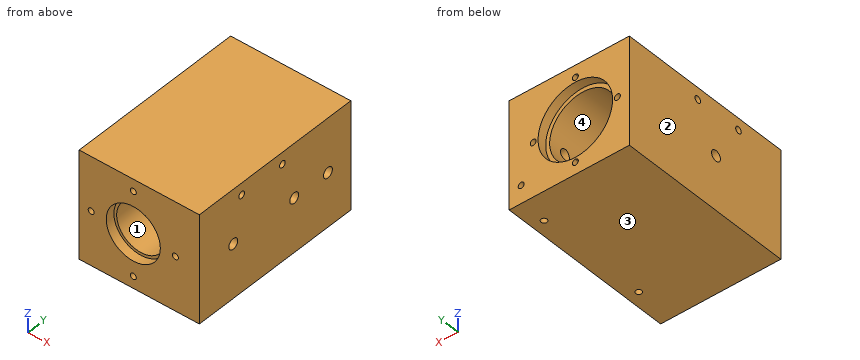
from build123d import *

# Parameters (mm, degrees)
F0_W      = 114.3
F0_H      = 114.3
F1_DEPTH  = 189.13856
F2_R      = 35.179
F3_DEPTH  = 96.52
F4_R      = 39.37
F5_DEPTH  = 9.525
F6_R      = 25.654
F7_DEPTH  = 71.12
F8_R      = 28.575
F9_DEPTH  = 9.525
F10_R     = 7.14375
F11_DEPTH = 118.01956
F12_R     = 5.55625
F13_DEPTH = 32.1059246971
F14_R     = 5.55625
F15_DEPTH = 52.6608720395
F16_DEPTH = 12.7
F18_R     = 3.175
F20_DEPTH = 52.6234315755
F19_R     = 3.175
F21_DEPTH = 146.7612
F24_DEPTH = 9.525
F25_R     = 3.175
F26_DEPTH = 9.525
F27_R     = 3.4925
F28_DEPTH = 127.0010001


with BuildPart() as f1:
    # F0 (on Front) → F1 (new body)
    with BuildSketch(Plane.XZ):
        Rectangle(F0_W, F0_H)
    extrude(amount=F1_DEPTH)

    # F2 (on face) → F3 (cut)
    with BuildSketch(Plane(origin=(0, 0, 0), x_dir=(-1, 0, 0), z_dir=(0, 1, 0))):
        Circle(F2_R)
    extrude(amount=-F3_DEPTH, mode=Mode.SUBTRACT)

    # F4 (on face) → F5 (cut)
    with BuildSketch(Plane(origin=(0, 0, 0), x_dir=(-1, 0, 0), z_dir=(0, 1, 0))):
        Circle(F4_R)
    extrude(amount=-F5_DEPTH, mode=Mode.SUBTRACT)

    # F6 (on face) → F7 (cut)
    with BuildSketch(Plane.XZ.offset(189.13856)):
        Circle(F6_R)
    extrude(amount=-F7_DEPTH, mode=Mode.SUBTRACT)

    # F8 (on face) → F9 (cut)
    with BuildSketch(Plane.XZ.offset(189.13856)):
        Circle(F8_R)
    extrude(amount=-F9_DEPTH, mode=Mode.SUBTRACT)

    # F10 (on face) → F11 (cut, through all)
    with BuildSketch(Plane.XZ.offset(118.01856)):
        Circle(F10_R)
    extrude(amount=-F11_DEPTH, mode=Mode.SUBTRACT)

    # F12 (on face) → F13 (cut, through all)
    with BuildSketch(Plane.YZ.offset(57.15)):
        with Locations((-146.80692, 0)):
            Circle(F12_R)
        with Locations((-70.69328, 0)):
            Circle(F12_R)
        with Locations((-28.575, 0)):
            Circle(F12_R)
    extrude(amount=-F13_DEPTH, mode=Mode.SUBTRACT)

    # F14 (on face) → F15 (cut, through all)
    with BuildSketch(Plane(origin=(-57.15, 0, 0), x_dir=(0, -1, 0), z_dir=(-1, 0, 0))):
        with Locations((108.17606, 0)):
            Circle(F14_R)
    extrude(amount=-F15_DEPTH, mode=Mode.SUBTRACT)

    # F16 (add): a face of the model
    f16_faces = [f1.faces().sort_by_distance(p)[0] for p in [
        (57.15, -94.7404141206, 0),
    ]]
    extrude(f16_faces, amount=F16_DEPTH)

    # F18 (on face) → F20 (cut, through all)
    with BuildSketch(Plane(origin=(0, 0, -57.15), x_dir=(1, 0, 0), z_dir=(0, 0, -1))):
        with Locations((57.15, 146.7612)):
            Circle(F18_R)
        with Locations((57.15, 28.575)):
            Circle(F18_R)
    extrude(amount=-F20_DEPTH, mode=Mode.SUBTRACT)

    # F19 (on face) → F21 (cut)
    with BuildSketch(Plane(origin=(0, 0, 0), x_dir=(-1, 0, 0), z_dir=(0, 1, 0))):
        with Locations((-57.15, -38.1)):
            Circle(F19_R)
    extrude(amount=-F21_DEPTH, mode=Mode.SUBTRACT)

    # F23 (on face) → F24 (cut)
    with BuildSketch(Plane.XZ):
        with BuildLine():
            ThreePointArc((-47.625, 0), (-44.45, -3.175), (-41.275, 0))
            Line((-41.275, 0), (-47.625, 0))
        make_face()
        with BuildLine():
            Line((-47.625, 0), (-41.275, 0))
            ThreePointArc((-41.275, 0), (-44.45, 3.175), (-47.625, 0))
        make_face()
        with BuildLine():
            ThreePointArc((41.275, 0), (44.45, -3.175), (47.625, 0))
            Line((47.625, 0), (41.275, 0))
        make_face()
        with BuildLine():
            Line((41.275, 0), (47.625, 0))
            ThreePointArc((47.625, 0), (44.45, 3.175), (41.275, 0))
        make_face()
        with BuildLine():
            ThreePointArc((0, -41.275), (-3.175, -44.45), (0, -47.625))
            Line((0, -47.625), (0, -41.275))
        make_face()
        with BuildLine():
            Line((0, -41.275), (0, -47.625))
            ThreePointArc((0, -47.625), (2.2450640303, -46.6950640303), (3.175, -44.45))
            ThreePointArc((3.175, -44.45), (2.2450640303, -42.2049359697), (0, -41.275))
        make_face()
        with BuildLine():
            ThreePointArc((0, 47.625), (-3.175, 44.45), (0, 41.275))
            Line((0, 41.275), (0, 47.625))
        make_face()
        with BuildLine():
            Line((0, 47.625), (0, 41.275))
            ThreePointArc((0, 41.275), (2.2450640303, 42.2049359697), (3.175, 44.45))
            ThreePointArc((3.175, 44.45), (2.2450640303, 46.6950640303), (0, 47.625))
        make_face()
    extrude(amount=F24_DEPTH, mode=Mode.SUBTRACT)

    # F25 (on face) → F26 (cut)
    with BuildSketch(Plane.XZ.offset(189.13856)):
        with Locations((-44.45, 0)):
            Circle(F25_R)
        with Locations((0, 44.45)):
            Circle(F25_R)
        with Locations((44.45, 0)):
            Circle(F25_R)
        with Locations((0, -44.45)):
            Circle(F25_R)
    extrude(amount=-F26_DEPTH, mode=Mode.SUBTRACT)

    # F27 (on face) → F28 (cut, through all)
    with BuildSketch(Plane.YZ.offset(69.85)):
        with Locations((-136.2554430962, 44.5877164602)):
            Circle(F27_R)
        with Locations((-85.4554430962, 44.5877164602)):
            Circle(F27_R)
    extrude(amount=-F28_DEPTH, mode=Mode.SUBTRACT)


solid = f1.part
The listing builds one solid part. Answer for the finished solid, in the listing's coordinates (mm). Face numbers are marked on the shaded views. Give positions to 0.01 mm unless a question says otherwise; leave off trailing zeros. Write each loop counter-clockwise with the first axis right and the second up, starting at its lowest first coordinate (ties: lowest second). Pieces come first, ordered by that corner, then holes. Notation, with made-up numbers: (2, -39.75) -> (21, -39.75) arc R5 ccw to (21, -33.75) -> close; hole circle Ø2 at (35, 60.5). An arc over 180 degrees is marked (long way). Use a Markdown table: item, result.
(1) Section B-B, the plane x = -22.5 is taken. Give the number of separate pieces and of enclosed holes in the cut face, then the cut area to 3 significant figures.
Return value:
| item | result |
|---|---|
| separate pieces | 1 |
| enclosed holes | 3 |
| area | 14,300 mm2 |
(2) Determine the mould class of the marked faces 1, 2, 3 and 4 for opening direction X: released by +X, released by -X, zero draft, split by the parting line, or undercut.
Return value:
| item | result |
|---|---|
| face 1 | undercut |
| face 2 | released by -X |
| face 3 | zero draft |
| face 4 | undercut |
(3) Section C-C, the plane z = 32 is taken. Determine the outline of the cut face in (x, y) (3 decimals).
Return value:
| item | result |
|---|---|
| outline | (-57.15, -189.139) -> (69.85, -189.139) -> (69.85, 0) -> (22.935, 0) -> (22.935, -9.525) -> (14.614, -9.525) -> (14.614, -96.52) -> (-14.614, -96.52) -> (-14.614, -9.525) -> (-22.935, -9.525) -> (-22.935, 0) -> (-57.15, 0) -> close |
(4) Section D-D, the plane y = -129.5 is taken. Determine the outline of the cut face in (x, z) (3 decimals), then the cut area to 3 significant figures.
Return value:
| item | result |
|---|---|
| outline | (-57.15, -57.15) -> (69.85, -57.15) -> (69.85, 57.15) -> (-57.15, 57.15) -> close; hole circle Ø51.308 at (0, 0); hole circle Ø6.35 at (57.15, -38.1) |
| area | 12,400 mm2 |
(5) Find the intervals of material crossed by probe 1 along Z at (x, y) = (0, -186) (3 decimals); probe 2 along Y at (x, z) = (57.15, -27.5); probe 3 along Z at (x, y) = (64.5, -147), in increasing order. Write a range as from..to.
Return value:
| item | result |
|---|---|
| probe 1 | -57.15..-47.625, -41.275..-28.575, 28.575..41.275, 47.625..57.15 |
| probe 2 | -189.14..-149.94, -143.59..-31.75, -25.4..0 |
| probe 3 | -57.15..-5.55, 5.55..57.15 |
(6) Section A-A, the plane y = -166.5 is taken. Determine the outline of the cut face in (x, z).
Return value:
| item | result |
|---|---|
| outline | (-57.15, -57.15) -> (69.85, -57.15) -> (69.85, 57.15) -> (-57.15, 57.15) -> close; hole circle Ø51.31 at (0, 0) |
(7) Flat-ended cylindrical pins translate along their axes: P1, Ø5, axis at x = 0, z = -44.5, coming from the -Y side; P2, Ø8, axis at y = -85.46, z = 44.59, coming from the +X side; P3, Ø1.9, axis at x = 1, z = -45, coming from the +Y side (3 decimals); P4, Ø21, axis at x = -0.5, z = 9, coming from the +Y side. Find the tip coordinate at first contact, or state that the pin passes through.
Return value:
| item | result |
|---|---|
| P1 | y = -179.61 |
| P2 | x = 69.85 |
| P3 | y = -9.525 |
| P4 | y = -96.52 |
